Check sheet for the drawn part. Datum: minimum x, y, z corner. Units: mm. A direction names the side the tool comes from. Coordinates: 2 decimals unless noted, no trailing zeros. Loops run counter-clockwise (first coordinate to the right, second up) from the corner with the lowest first, then second, coordinate; pieces in that order, holes last.
Q1. Access from +Z, -Z, +X, -X, +Y, -Y to the whole of each face (thin tool, end or side, straight path). Record for the marked faces 1, 2 and 3.
Q2. Mould release check, pull along Y, two halves, no side actions. Record for the marked faces 4, 5 and 6: +Y half, -Y half, draft (parallel to the pull), parting line (faces both ways), or undercut.
Q3. Sectioned sample at B-B (x = 116). Enter the section's corners in (y, z), then the cut area to 3 significant figures.
Q4. Go/stop test with flat-tipped pins: P1, Ø5, axis at x = 182, y = 115.5, coming from the -Z side; P2, Ø15, axis at y = 69.5, z = 56, coming from the -X side; P3, Ø5, axis at x = 148.5, y = 211.5, coming from the +Z side; P4, Ø1, axis at x = 110.5, y = 228, coming from the -Z side. Record where each tip stops, or that it passes through.
Q5. Sectioned sample at C-C (z = 53.5). Enter the section's corners in (x, y).
Q6. Sectioned sample at D-D (x = 149.5). Enter the section's corners in (y, z).
Q7. Material ranges on probe 1 along Y at (x, z) = (72.5, 50.5); probe 2 along X at (y, z) = (148.5, 67); probe 3 along Y at (x, z) = (66, 100), recorded low to high.
Q8. Sectioned sample at A-A (y = 91). Enter the section's corners in (x, z), then the cut area to 3 significant figures.
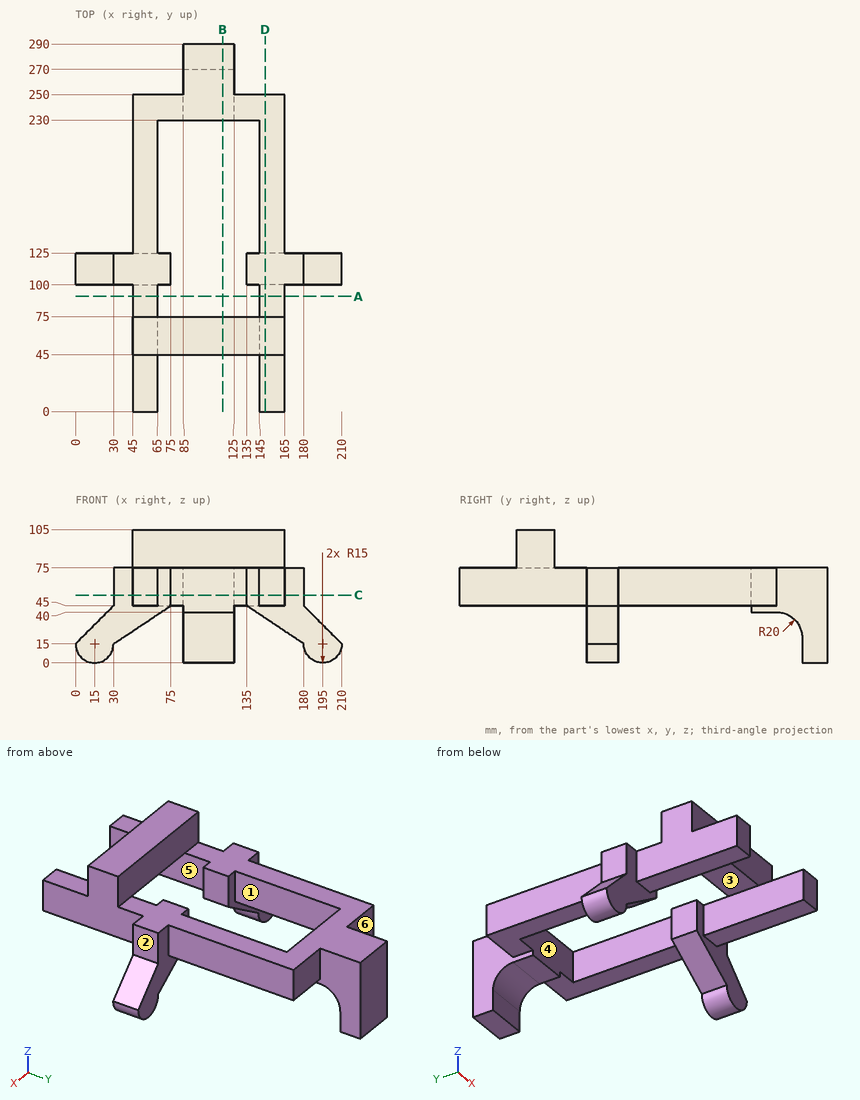
Geometry check:
1. face 1: +Z, -Z
1. face 2: +Z, +X, +Y, -Y
1. face 3: -Z, -Y
2. face 4: undercut
2. face 5: draft
2. face 6: +Y half
3. outline: (45, 75) - (75, 75) - (75, 105) - (45, 105) - close; (230, 40) - (250, 40) arc R20 cw to (270, 20) - (270, 0) - (290, 0) - (290, 75) - (230, 75) - close
3. area: 3,890 mm2
4. P1: stops at z = 4.29
4. P2: stops at x = 45
4. P3: stops at z = 75
4. P4: passes through
5. outline: (30, 100) - (45, 100) - (45, 0) - (65, 0) - (65, 100) - (75, 100) - (75, 125) - (65, 125) - (65, 230) - (145, 230) - (145, 125) - (135, 125) - (135, 100) - (145, 100) - (145, 0) - (165, 0) - (165, 100) - (180, 100) - (180, 125) - (165, 125) - (165, 250) - (125, 250) - (125, 290) - (85, 290) - (85, 250) - (45, 250) - (45, 125) - (30, 125) - close
6. outline: (0, 45) - (100, 45) - (100, 35.33) - (125, 35.33) - (125, 45) - (250, 45) - (250, 75) - (75, 75) - (75, 105) - (45, 105) - (45, 75) - (0, 75) - close
7. probe 1: y = 100 to 125, 230 to 250
7. probe 2: x = 45 to 65, 145 to 165
7. probe 3: y = 45 to 75
8. outline: (45, 45) - (65, 45) - (65, 75) - (45, 75) - close; (145, 45) - (165, 45) - (165, 75) - (145, 75) - close
8. area: 1,200 mm2
